The model under review builds one solid part; all positions refer to its coordinate system, in mm. A direction names the side the tool comes from. Round coordinates to 2 decimals unless told otherwise and drop trailing zeros. Order: outer loops, then holes, each group sorted by start corner. A loop starts at its lowest first (then second) coordinate and runs counter-clockwise, first axis right, second up.
```python
from build123d import *

# Parameters (mm, degrees)
MODEL_W                  = 79.9
MODEL_H                  = 48.698269882
MODEL_R                  = 1.8
MODEL_W_2                = 6.8
MODEL_H_2                = 13.312275424
MODEL_W_3                = 6.6
MODEL_H_3                = 7
MODEL_W_4                = 49.999979697
MODEL_H_4                = 10.999995003
RESSALTO_EXTRUS_O1_DEPTH = 6


with BuildPart() as part:
    # Model → Ressalto-extrusão1 (new body)
    with BuildSketch(Plane.XY):
        with Locations((70.266607808, 31.590543985)):
            Rectangle(MODEL_W, MODEL_H)
        with Locations((53.816607808, 11.757142514)):
            Circle(MODEL_R, mode=Mode.SUBTRACT)
        with Locations((92.766607808, 50.939678926)):
            Circle(MODEL_R, mode=Mode.SUBTRACT)
        with Locations((86.716607808, 11.757142514)):
            Circle(MODEL_R, mode=Mode.SUBTRACT)
        with Locations((47.766607808, 50.939678926)):
            Circle(MODEL_R, mode=Mode.SUBTRACT)
        with Locations((40.316607808, 17.595816638)):
            Rectangle(MODEL_W_2, MODEL_H_2, mode=Mode.SUBTRACT)
        with Locations((40.416607808, 47.639678926)):
            Rectangle(MODEL_W_3, MODEL_H_3, mode=Mode.SUBTRACT)
        with Locations((100.216607808, 17.595816638)):
            Rectangle(MODEL_W_2, MODEL_H_2, mode=Mode.SUBTRACT)
        with Locations((100.216607808, 47.639678926)):
            Rectangle(MODEL_W_2, MODEL_H_3, mode=Mode.SUBTRACT)
        with Locations((70.266607808, 33.557142515)):
            Rectangle(MODEL_W_4, MODEL_H_4, mode=Mode.SUBTRACT)
    extrude(amount=RESSALTO_EXTRUS_O1_DEPTH)


solid = part.part
```
(1) Consider section D-D (y = 36). Write out the cut boundary in (x, z).
Data:
outline: (30.32, 0) - (45.27, 0) - (45.27, 6) - (30.32, 6) - close; (95.27, 0) - (110.22, 0) - (110.22, 6) - (95.27, 6) - close
(2) Consider section A-A (y = 18). Write out the cut boundary in (x, z).
Data:
outline: (30.32, 0) - (36.92, 0) - (36.92, 6) - (30.32, 6) - close; (43.72, 0) - (96.82, 0) - (96.82, 6) - (43.72, 6) - close; (103.62, 0) - (110.22, 0) - (110.22, 6) - (103.62, 6) - close
(3) Consider section C-C (x = 57). Write out the cut boundary in (y, z).
Data:
outline: (7.24, 0) - (28.06, 0) - (28.06, 6) - (7.24, 6) - close; (39.06, 0) - (55.94, 0) - (55.94, 6) - (39.06, 6) - close
(4) For faces 5 (the flat face through (70, 28.057, 3)), 6 (the flat face through (70, 7.241, 3)), list the 3-axis set-ups (+Z, -Z, +X, -X, +Y, -Y) from which the entire face can be reached by the end or side of a thin tool; tool diameter is ignored.
Data:
face 5: +Z, -Z
face 6: +Z, -Z, +X, -X, -Y
(5) Draft analysis for pull direction X (two halves, no side actions). For faces 1 (the flat face through (40, 44.14, 3)), 2 (the flat face through (100, 10.94, 3)), 3 (the flat face through (110.217, 31, 3)), 4 (the flat face through (70, 27, 6)), state which applies: pulls with the +X half, pulls with the -X half, needs draft (parallel to the pull), parting line crosses it, or undercut.
Data:
face 1: undercut
face 2: undercut
face 3: pulls with the +X half
face 4: needs draft
(6) Consider section B-B (x = 42). Write out the cut boundary in (y, z), and give its area (3 significant figures).
Data:
outline: (7.24, 0) - (10.94, 0) - (10.94, 6) - (7.24, 6) - close; (24.25, 0) - (44.14, 0) - (44.14, 6) - (24.25, 6) - close; (51.14, 0) - (55.94, 0) - (55.94, 6) - (51.14, 6) - close
area: 170 mm2
(7) To check wall thickness, follow probe 1 along X at (y, z) = (22.5, 1.75); probe 2 along X at (y, z) = (47, 2.4); probe 3 along Y at (x, z) = (41, 2.9). State the ranges of each line that lie inside material, in increasing order.
Data:
probe 1: x = 30.32 to 36.92, 43.72 to 96.82, 103.62 to 110.22
probe 2: x = 30.32 to 37.12, 43.72 to 96.82, 103.62 to 110.22
probe 3: y = 7.24 to 10.94, 24.25 to 44.14, 51.14 to 55.94
